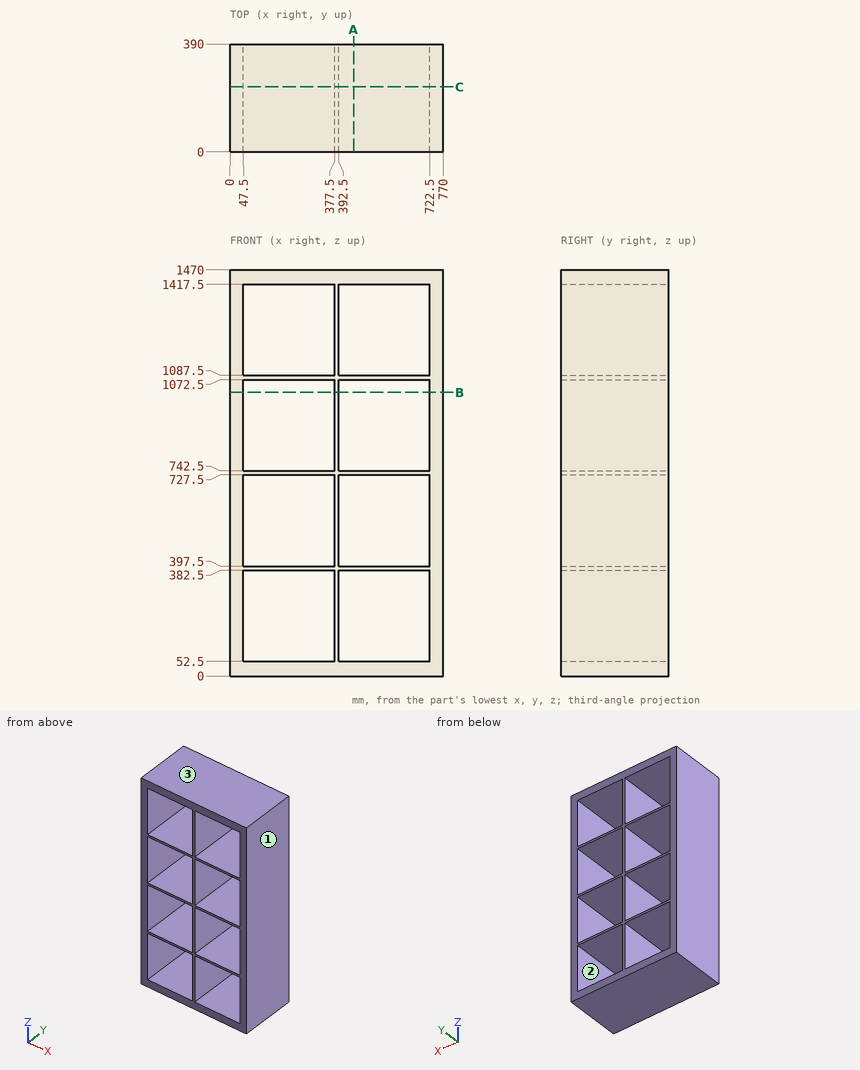
The drawing under review shows one solid part. Ordinate dimensions are in mm from its lowest x, y, z. Round coordinates to 2 decimals unless told otherwise and drop trailing zeros. Loops run counter-clockwise (first coordinate to the right, second up) from the corner with the lowest first, then second, coordinate; pieces in that order, holes last. Notation, with made-up numbers: (-13, 69.5) - (31, 69.5) arc R24 cw to (31, 93.5) - close; hole circle Ø5 at (85.25, 7.5). An arc over 180 degrees is marked (long way). Use a Markdown table: item, result. Add a question column.
Q1. Add section B-B (z = 1026). State the section outline as (x, y) points, plus the area to 3 significant figures.
Q2. For probe 1 along Z at (x, y) = (137.5, 214); probe 2 along X at (y, z) = (130.5, 1066), list the stretches that pass through material, from the lowest coordinate up.
Q3. Add section C-C (y = 234.5). State how many separate pieces and enclosed holes the cut face has, plus the area to 3 significant figures.
Q4. The part is to be moulded in two halves that separate along Z. For the marked faces 1, 2 and 3, say which applies: pulls with the +Z half, pulls with the -Z half, needs draft (parallel to the pull), parting line crosses it, or undercut.
Q5. Add section A-A (x = 446.5). State the section outline as (y, z) points.
Worked answers:
| question | item | result |
|---|---|---|
| 1 | outline | (0, 0) - (47.5, 0) - (47.5, 390) - (0, 390) - close; (377.5, 0) - (392.5, 0) - (392.5, 390) - (377.5, 390) - close; (722.5, 0) - (770, 0) - (770, 390) - (722.5, 390) - close |
| 1 | area | 42,900 mm² |
| 2 | probe 1 | 0 to 52.5, 382.5 to 397.5, 727.5 to 742.5, 1072.5 to 1087.5, 1417.5 to 1470 |
| 2 | probe 2 | 0 to 47.5, 377.5 to 392.5, 722.5 to 770 |
| 3 | separate pieces | 1 |
| 3 | enclosed holes | 8 |
| 3 | area | 261,000 mm² |
| 4 | face 1 | needs draft |
| 4 | face 2 | undercut |
| 4 | face 3 | pulls with the +Z half |
| 5 | outline | (0, 0) - (390, 0) - (390, 52.5) - (0, 52.5) - close; (0, 382.5) - (390, 382.5) - (390, 397.5) - (0, 397.5) - close; (0, 727.5) - (390, 727.5) - (390, 742.5) - (0, 742.5) - close; (0, 1072.5) - (390, 1072.5) - (390, 1087.5) - (0, 1087.5) - close; (0, 1417.5) - (390, 1417.5) - (390, 1470) - (0, 1470) - close |
